Geometry: see drawing. Coordinates: mm, zero at the bounding-box minimum. Coordinates: 2 decimals unless noted, no trailing zeros. Loops run counter-clockwise (first coordinate to the right, second up) from the corner with the lowest first, then second, coordinate; pieces in that order, holes last.
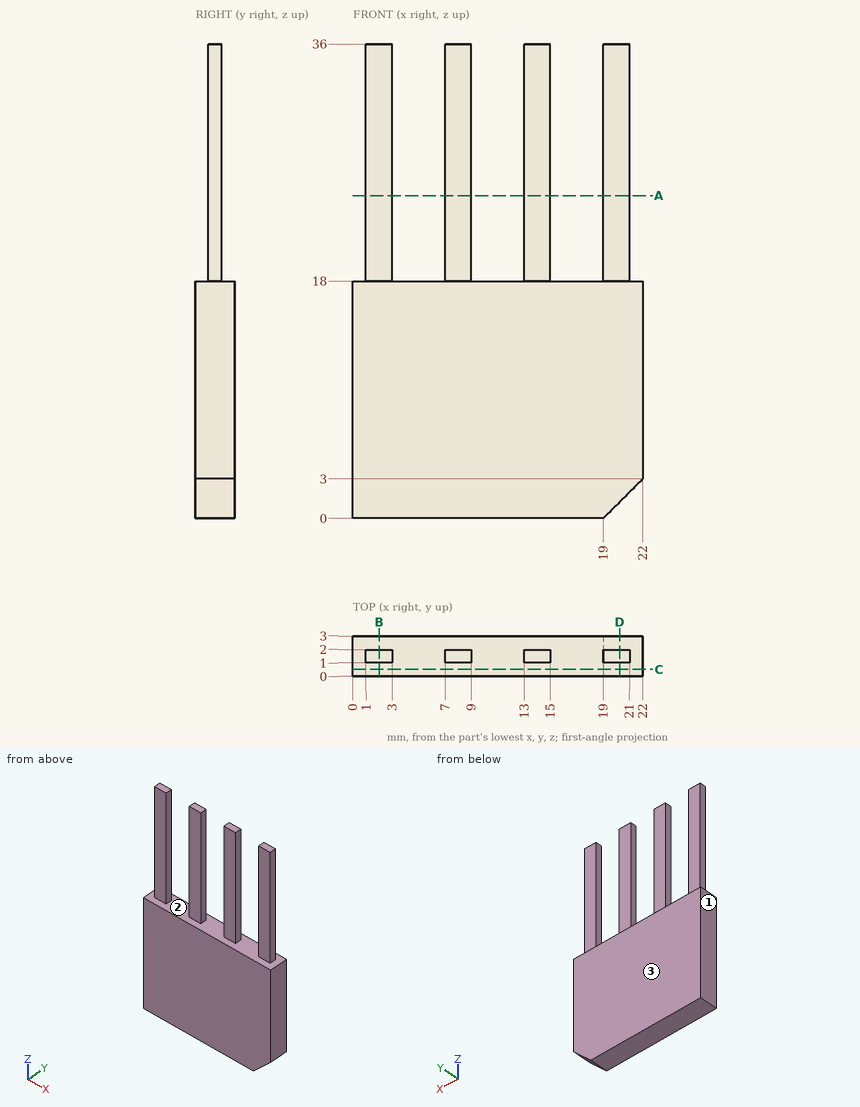
Item 1: Mould query, pull axis X, two halves, no side actions, for the marked faces 1, 2 and 3. Classes: +X half, -X half, draft (parallel to the pull), parting line (faces both ways), or undercut.
Result:
face 1: -X half
face 2: undercut
face 3: draft
Item 2: Section query D-D (x = 20.25). Output: boundary loops of the cut face in (y, z), then the cut area to 4 significant figures.
Result:
outline: (0, 1.25) - (3, 1.25) - (3, 18) - (2, 18) - (2, 36) - (1, 36) - (1, 18) - (0, 18) - close
area: 68.25 mm2
Item 3: Section query A-A (z = 24.5). Output: boundary loops of the cut face in (x, y).
Result:
outline: (1, 1) - (3, 1) - (3, 2) - (1, 2) - close; (7, 1) - (9, 1) - (9, 2) - (7, 2) - close; (13, 1) - (15, 1) - (15, 2) - (13, 2) - close; (19, 1) - (21, 1) - (21, 2) - (19, 2) - close
Item 4: Section query C-C (y = 0.5). Output: boundary loops of the cut face in (x, z).
Result:
outline: (0, 0) - (19, 0) - (22, 3) - (22, 18) - (0, 18) - close
Item 5: Line query: L1, parallel to X at y = 1.15, z = 19; L2, parallel to Z at x = 4.75, y = 0.45; L3, parallel to Y at x = 7.5, z = 32. Output: solid intervals per line, ascending.
Result:
L1: x = 1 to 3, 7 to 9, 13 to 15, 19 to 21
L2: z = 0 to 18
L3: y = 1 to 2
Item 6: Section query B-B (x = 2). Output: boundary loops of the cut face in (y, z).
Result:
outline: (0, 0) - (3, 0) - (3, 18) - (2, 18) - (2, 36) - (1, 36) - (1, 18) - (0, 18) - close
Item 7: Contact query for flat-ended pins moving along their axis: P1, Ø1, axis at x = 7.5, z = 26.5, coming from the -Y side; P2, Ø1.6, axis at x = 14.5, z = 31, coming from the +Y side; P3, Ø0.8, axis at y = 1.5, z = 25, coming from the +X side. Output: stop coordinate, or through.
Result:
P1: stops at y = 1
P2: stops at y = 2
P3: stops at x = 21
